Read the model definition and answer for the solid it produces. Units are mm, in the model's axes. A direction names the side the tool comes from. Give positions to 0.01 mm unless a question says otherwise; leave off trailing zeros. Write each loop counter-clockwise with the first axis right and the second up, starting at its lowest first coordinate (ties: lowest second). Pieces come first, ordered by that corner, then holes. Notation, with made-up numbers: M 30,36.25 L 51,36.25 A19 cw 51,58.25 Z; hole C 77.5,37 d4. An arc over 180 degrees is marked long. Use a Markdown table: item, result. Add a question column.
Item 1: Given P1, Ø2, axis at x = -12, z = 11, coming from the +Y side; P2, Ø1, axis at x = -5, z = -2.5, coming from the +Y side; P3, Ø5, axis at x = -24.13, z = 11.94, coming from the +Y side, each flat-ended and moving along its own axis, determine where each tip first touches the part or whether it passes through.
Item 2: For faces 1 (the cylindrical face through (-15.778, 6.297, 17.293)), 2 (the cylindrical face through (-22.611, 1.878, 13.594)), determine the directions among +Z, -Z, +X, -X, +Y, -Y from which every point of the face is accessible in a straight line to the end or side of a thin tool.
Item 3: The mould has two halves that part along X. Classify faces 3 (the flat face through (19.05, 5, 0)), 4 (the flat face through (0, 6, 17.78)), 5 (the flat face through (-18, 10.16, 1)): pulls with the +X half, pulls with the -X half, needs draft (parallel to the pull), parting line crosses it, or undercut.
Item 4: A cutting plane is placed at B-B on x = -24.13. Determine the outline of the cut face in (y, z).
Item 5: Consider probe 1 along X at (y, z) = (9.5, 13.5); probe 2 along Z at (x, y) = (16.5, 8.25). Determine where each line is inside the solid, lowest interval first. Write a range as [from, to].
Item 6: A cutting plane is placed at C-C on y = 1.5. Determine the outline of the cut face in (x, z), then the cut area to 3 significant figures.
Item 7: A cutting plane is placed at A-A on y = 4.5. Count the separate pieces of the cut face and the enclosed holes in it, then the cut area to 3 significant figures.
Item 8: A cutting plane is placed at D-D on z = 11. Determine the outline of the cut face in (x, y).
from build123d import *

# Parameters (mm, degrees)
SKETCH1_W           = 38.1
SKETCH1_H           = 38.1
BOSS_EXTRUDE1_DEPTH = 2.54
SKETCH2_W           = 38.1
SKETCH2_H           = 38.1
SKETCH2_R           = 1.27
BOSS_EXTRUDE2_DEPTH = 7.62
SKETCH4_R           = 3.030246623
SKETCH4_R_2         = 0.88307969
SKETCH4_W           = 2.032
SKETCH4_H           = 2.032
BOSS_EXTRUDE3_DEPTH = 2.54
SKETCH7_W           = 10.16
SKETCH7_H           = 38.1
SKETCH7_R           = 2.2479
BOSS_EXTRUDE5_DEPTH = 3.81


with BuildPart() as part:
    # Sketch1 → Boss-Extrude1 (new body)
    with BuildSketch(Plane(origin=(0, 0, 0), x_dir=(1, 0, 0), z_dir=(0, 1, 0))):
        Rectangle(SKETCH1_W, SKETCH1_H)
    extrude(amount=BOSS_EXTRUDE1_DEPTH)

    # Sketch2 → Boss-Extrude2 (add)
    # profile 1 of 2: a face of its own
    with BuildSketch(Plane(origin=(0, 2.54, 0), x_dir=(1, 0, 0), z_dir=(0, 1, 0))):
        Rectangle(SKETCH2_W, SKETCH2_H)
        with Locations(Location((-17.018, -17.018, 0), (0, 0, 90))):
            Circle(SKETCH2_R, mode=Mode.SUBTRACT)
        with Locations(Location((17.018, -17.018, 0), (0, 0, 90))):
            Circle(SKETCH2_R, mode=Mode.SUBTRACT)
        with BuildLine():
            Line((14.940193669, 15.24), (15.24, 15.24))
            Line((15.24, 15.24), (15.24, 14.940193669))
            ThreePointArc((15.24, 14.940193669), (16.420507838, 14.220803312), (17.78, 13.97))
            Line((17.78, 13.97), (17.78, -13.97))
            ThreePointArc((17.78, -13.97), (15.085923164, -15.085923164), (13.97, -17.78))
            Line((13.97, -17.78), (-13.97, -17.78))
            ThreePointArc((-13.97, -17.78), (-15.085923164, -15.085923164), (-17.78, -13.97))
            Line((-17.78, -13.97), (-17.78, 13.97))
            ThreePointArc((-17.78, 13.97), (-15.085923164, 15.085923164), (-13.97, 17.78))
            Line((-13.97, 17.78), (13.97, 17.78))
            ThreePointArc((13.97, 17.78), (14.220803312, 16.420507838), (14.940193669, 15.24))
        make_face(mode=Mode.SUBTRACT)
        with Locations(Location((-17.018, 17.018, 0), (0, 0, 90))):
            Circle(SKETCH2_R, mode=Mode.SUBTRACT)
        with Locations(Location((17.018, 17.018, 0), (0, 0, 90))):
            Circle(SKETCH2_R, mode=Mode.SUBTRACT)
    # profile 2 of 2: a face of its own
    with BuildSketch(Plane(origin=(0, 2.54, 0), x_dir=(1, 0, 0), z_dir=(0, 1, 0))):
        with BuildLine():
            Line((15.24, 14.940193669), (15.24, 15.24))
            Line((15.24, 15.24), (14.940193669, 15.24))
            ThreePointArc((14.940193669, 15.24), (15.085923164, 15.085923164), (15.24, 14.940193669))
        make_face()
    extrude(amount=BOSS_EXTRUDE2_DEPTH)

    # Sketch4 → Boss-Extrude3 (add)
    # profile 1 of 3: a face of its own
    with BuildSketch(Plane(origin=(0, 2.54, 0), x_dir=(1, 0, 0), z_dir=(0, 1, 0))):
        with Locations(Location((0, 10.947233516, 0), (0, 0, 270))):
            Circle(SKETCH4_R)
        with Locations(Location((0, 10.947233516, 0), (0, 0, 270))):
            Circle(SKETCH4_R_2, mode=Mode.SUBTRACT)
    # profile 2 of 3: a face of its own
    with BuildSketch(Plane(origin=(0, 2.54, 0), x_dir=(1, 0, 0), z_dir=(0, 1, 0))):
        with Locations((-12.16137027, -11.201233516)):
            Rectangle(SKETCH4_W, SKETCH4_H)
    # profile 3 of 3: a face of its own
    with BuildSketch(Plane(origin=(0, 2.54, 0), x_dir=(1, 0, 0), z_dir=(0, 1, 0))):
        with Locations((11.557, -11.201233516)):
            Rectangle(SKETCH4_W, SKETCH4_H)
    extrude(amount=BOSS_EXTRUDE3_DEPTH)

    # Sketch7 → Boss-Extrude5 (add)
    with BuildSketch(Plane.XZ):
        with Locations((-24.13, 0)):
            Rectangle(SKETCH7_W, SKETCH7_H)
        with Locations(Location((-24.13, -10.990632384, 0), (0, 0, 270))):
            Circle(SKETCH7_R, mode=Mode.SUBTRACT)
        with Locations(Location((-24.13, 11.937008295, 0), (0, 0, 270))):
            Circle(SKETCH7_R, mode=Mode.SUBTRACT)
    extrude(amount=-BOSS_EXTRUDE5_DEPTH)


solid = part.part
Filled in:
| question | item | result |
|---|---|---|
| 1 | P1 | y = 5.08 |
| 1 | P2 | y = 2.54 |
| 1 | P3 | y = 3.81 |
| 2 | face 1 | +Y |
| 2 | face 2 | +Y, -Y |
| 3 | face 3 | pulls with the +X half |
| 3 | face 4 | undercut |
| 3 | face 5 | needs draft |
| 4 | outline | M 0,-19.05 L 3.81,-19.05 L 3.81,-13.24 L 0,-13.24 Z; M 0,-8.74 L 3.81,-8.74 L 3.81,9.69 L 0,9.69 Z; M 0,14.18 L 3.81,14.18 L 3.81,19.05 L 0,19.05 Z |
| 5 | probe 1 | [-19.05, -17.78], [17.78, 19.05] |
| 5 | probe 2 | [-19.05, -18.18], [-15.86, -14.19], [14.19, 15.86], [18.18, 19.05] |
| 6 | outline | M -29.21,-19.05 L 19.05,-19.05 L 19.05,19.05 L -29.21,19.05 Z; hole C -24.13,-10.99 d4.5; hole C -24.13,11.94 d4.5 |
| 6 | area | 1,810 mm² |
| 7 | separate pieces | 4 |
| 7 | enclosed holes | 6 |
| 7 | area | 247 mm² |
| 8 | outline | M -29.21,0 L -26.17,0 L -26.17,3.81 L -29.21,3.81 Z; M -22.09,0 L 19.05,0 L 19.05,10.16 L 17.78,10.16 L 17.78,2.54 L 12.57,2.54 L 12.57,5.08 L 10.54,5.08 L 10.54,2.54 L -11.15,2.54 L -11.15,5.08 L -13.18,5.08 L -13.18,2.54 L -17.78,2.54 L -17.78,10.16 L -19.05,10.16 L -19.05,3.81 L -22.09,3.81 Z |
